Can you work these out from the model? Positions are in its coordinate system, mm. Face numbers are marked on the shaded views. Give positions to 0.01 mm unless a question says otherwise; leave off trailing zeros. Write each loop counter-clockwise with the first axis right and the second up, starting at its lowest first coordinate (ties: lowest second). Pieces come first, ordered by that corner, then holes. Notation, with made-up numbers: M 74,44.5 L 89,44.5 A28 cw 89,68.5 Z; hole C 60,59 d2. An arc over 180 degrees is marked long. Write each question's results on one line, items separated by ' | '.
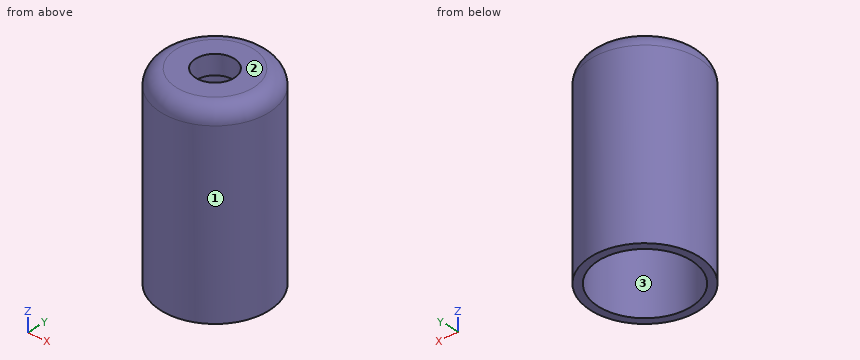
from build123d import *

# Parameters (mm, degrees)
SKETCH_R        = 7
PAD_DEPTH       = 25
SKETCH002_R     = 6
POCKET_DEPTH    = 22.5
SKETCH001_R     = 2.5
POCKET001_DEPTH = 3
FILLET_R        = 2


with BuildPart() as part:
    # Sketch → Pad (new body)
    with BuildSketch(Plane.XY):
        Circle(SKETCH_R)
    extrude(amount=PAD_DEPTH)

    # Sketch002 → Pocket (cut)
    with BuildSketch(Plane(origin=(0, 0, 0), x_dir=(1, 0, 0), z_dir=(0, 0, -1))):
        Circle(SKETCH002_R)
    extrude(amount=-POCKET_DEPTH, mode=Mode.SUBTRACT)

    # Sketch001 (on Face3 of Pad) → Pocket001 (cut)
    with BuildSketch(Plane.XY.offset(25)):
        Circle(SKETCH001_R)
    extrude(amount=-POCKET001_DEPTH, mode=Mode.SUBTRACT)

    # Fillet
    fillet_edges = [part.edges().sort_by_distance(p)[0] for p in [
        (-7, 0, 25),
    ]]
    fillet(fillet_edges, radius=FILLET_R)


solid = part.part
Item 1: If I drill on line 1 (Y direction, x = 0, z = 14); line 2 (X direction, y = 0.25, z = 13.25); line 3 (Y direction, x = 2, z = 9), over which ranges is the centre line in solid material (lowest first)? Write a range as from..to.
Geometry says:
line 1: y = -7..-6, 6..7 | line 2: x = -7..-5.99, 5.99..7 | line 3: y = -6.71..-5.66, 5.66..6.71
Item 2: I'm going to push flat-ended pins straight in: pin 1 (7 mm diameter, centred on x = 0, y = 0, fed in from -Z); pin 2 (5 mm diameter, centred on x = -2, y = -5, fed in from -Z); pin 3 (1 mm diameter, centred on x = -2.5, z = 13.5, fed in from +Y); pin 4 (1.5 mm diameter, centred on y = -2.5, z = 8.5, fed in from -X). Where does each tip first touch, or does it pass through?
Geometry says:
pin 1: stops at z = 22.5 | pin 2: stops at z = 0 | pin 3: stops at y = 6.71 | pin 4: stops at x = -6.78
Item 3: I want a section at A-A, the plane x = 0. Please give me the cut outline in (y, z), and give its area (3 significant figures).
Geometry says:
outline: M -7,0 L -6,0 L -6,22.5 L -2.5,22.5 L -2.5,25 L -5,25 A2 ccw -7,23 Z; M 2.5,22.5 L 6,22.5 L 6,0 L 7,0 L 7,23 A2 ccw 5,25 L 2.5,25 Z | area: 65.8 mm2
Item 4: Thinking about a two-plate mould opening in X: for the marked faces 1, 2 and 3, which applies, +X half, -X half, draft (parallel to the pull), parting line (faces both ways), or undercut?
Geometry says:
face 1: parting line | face 2: draft | face 3: undercut
Item 5: I want a section at C-C, the plane z = 13.5. Please give me the cut outline in (x, y).
Geometry says:
outline: C 0,0 d14; hole C 0,0 d12
